from build123d import *

# Parameters (mm, degrees)
SKETCH1_R           = 4
BOSS_EXTRUDE1_DEPTH = 10


with BuildPart() as part:
    # Sketch1 → Boss-Extrude1 (new body)
    with BuildSketch(Plane(origin=(0, 0, 0), x_dir=(1, 0, 0), z_dir=(0, 1, 0))):
        with BuildLine():
            Line((-2.88, 7.463618425), (40.64, 24.256759883))
            ThreePointArc((40.64, 24.256759883), (75.371520283, 5.682073435), (51.88, -25.931941694))
            ThreePointArc((51.88, -25.931941694), (56.44926926, -13.322161987), (58, 0))
            ThreePointArc((58, 0), (50, 8), (42, 0))
            ThreePointArc((42, 0), (40.364821154, -11.60522353), (35.586608897, -22.306798678))
            Line((35.586608897, -22.306798678), (-2.88, -7.463618425))
            ThreePointArc((-2.88, -7.463618425), (-8, 0), (-2.88, 7.463618425))
        make_face()
        with Locations(Location((0, 0, 0), (0, 0, 270))):
            Circle(SKETCH1_R, mode=Mode.SUBTRACT)
    extrude(amount=BOSS_EXTRUDE1_DEPTH)


solid = part.part
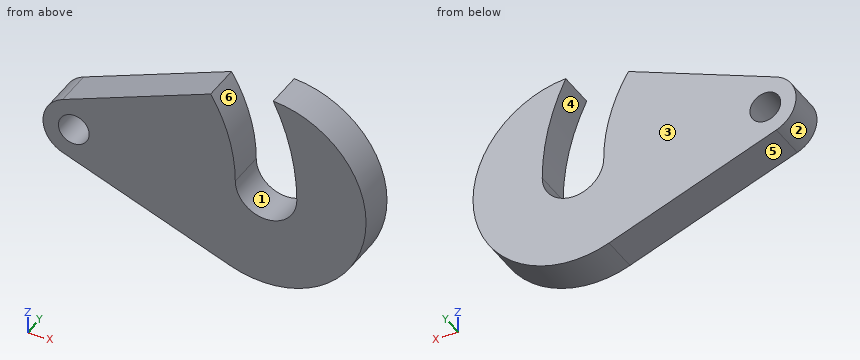
The model under review builds one solid part; all positions refer to its coordinate system, in mm. Face numbers are marked on the shaded views. A direction names the side the tool comes from. Round coordinates to 2 decimals unless told otherwise and drop trailing zeros. Order: outer loops, then holes, each group sorted by start corner. A loop starts at its lowest first (then second) coordinate and runs counter-clockwise, first axis right, second up. Notation, with made-up numbers: (43, 56) - (58, 56) arc R29 ccw to (58, 81) - close; hole circle Ø6 at (45.25, 58.5). An arc over 180 degrees is marked (long way). Use one line per item in the form item = value.
Q1. Add section A-A on y = 9. Give the boundary of the cut face in (x, z).
Response values:
outline = (-2.88, -7.46) - (40.64, -24.26) arc R26 ccw (long way) to (51.88, 25.93) arc R58 cw to (58, 0) arc R8 cw to (42, 0) arc R42 ccw to (35.59, 22.31) - (-2.88, 7.46) arc R8 ccw to start; hole circle Ø8 at (0, 0)
Q2. Add section C-C on x = 0. Give the boundary of the cut face in (y, z).
Response values:
outline = (0, -8.57) - (10, -8.57) - (10, -4) - (0, -4) - close; (0, 4) - (10, 4) - (10, 8.57) - (0, 8.57) - close
Q3. Tool access review of the marked faces 4, 5 and 6: name each direction out of +Z, -Z, +X, -X, +Y, -Y from which nothing blocks a thin tool from reaching the whole face with its end or side.
Response values:
face_4 = +Y, -Y
face_5 = -Z, -X, +Y, -Y
face_6 = +Z, +Y, -Y
Q4. Clearance check with flat-ended pins moving along their axes: P1, Ø2, axis at x = 37.5, y = 6, coming from the +Z side; P2, Ø1, axis at y = 3, z = -1, coming from the +X side; P3, Ø5, axis at y = 2.5, z = -9.5, coming from the -X side; P4, Ø5, axis at x = 0, z = 0, coming from the +Y side. State where each tip first meets the part, or that it passes through.
Response values:
P1 = 20.78
P2 = 76
P3 = -3.87
P4 = through
Q5. Add section B-B on z = 19. Give the boundary of the cut face in (x, y), then the cut area to 3 significant figures.
Response values:
outline = (27.02, 0) - (37.46, 0) - (37.46, 10) - (27.02, 10) - close; (54.8, 0) - (67.75, 0) - (67.75, 10) - (54.8, 10) - close
area = 234 mm^2
Q6. Add section D-D on x = 50. Give the boundary of the cut face in (y, z).
Response values:
outline = (0, -26) - (10, -26) - (10, -8) - (0, -8) - close
Q7. To check wall thickness, follow line 1 (X direction, y = 5.5, z = 0); line 2 (X direction, y = 3, z = 1); line 3 (Z direction, x = -3.5, y = 6.5). State the ranges of each line that lie inside material, in increasing order.
Response values:
line_1 = -8 to -4, 4 to 42, 58 to 76
line_2 = -7.94 to -3.87, 3.87 to 41.99, 57.99 to 75.98
line_3 = -7.19 to -1.94, 1.94 to 7.19
Q8. Mouldability with a two-part tool opening along X and no side actions: class the marked faces 1, 2 and 3 as pulls with the +X half, pulls with the -X half, needs draft (parallel to the pull), parting line crosses it, or undercut.
Response values:
face_1 = undercut
face_2 = pulls with the -X half
face_3 = needs draft
